Can you work these out from the model? Positions are in its coordinate system, mm. Give positions to 0.01 mm unless a question says otherwise; leave off trailing zeros. Loops run counter-clockwise (first coordinate to the right, second up) from the corner with the lowest first, then second, coordinate; pieces in that order, holes last. Notation, with made-up numbers: M -40,19 L -30,19 A24 ccw -30,57 Z; hole C 84,-17 d2. An arc over 180 degrees is marked long. Put each result on its own line as item: value. Start each with the question number.
1) Imagine slicing it at A-A (x = 231.5). Write out the boundary of the cut face in (y, z), then the cut area to 3 significant figures.
2) Please list where these lines run through material, in increasing order: line 1 along Z through (x, y) = (548, 40); line 2 along Z through (x, y) = (228, 70); line 3 along Y through (x, z) = (638, 6.5). Write a range as from..to.
3) Imagine slicing it at B-B (y = 31.5). Write out the boundary of the cut face in (x, z), then the cut area to 3 significant figures.
4) For P1, Ø5, axis at x = 317, y = 3, coming from the +Z side; P2, Ø6.5, axis at x = 681.5, z = 5, coming from the -Y side; P3, Ø6.5, axis at y = 66, z = 7.5, coming from the +X side, each with a flat end and sliding along its axis, tell me the tip position at first contact or that it passes through.
5) Imagine slicing it at C-C (z = 2.5). Write out the boundary of the cut face in (x, y), then the cut area to 3 significant figures.
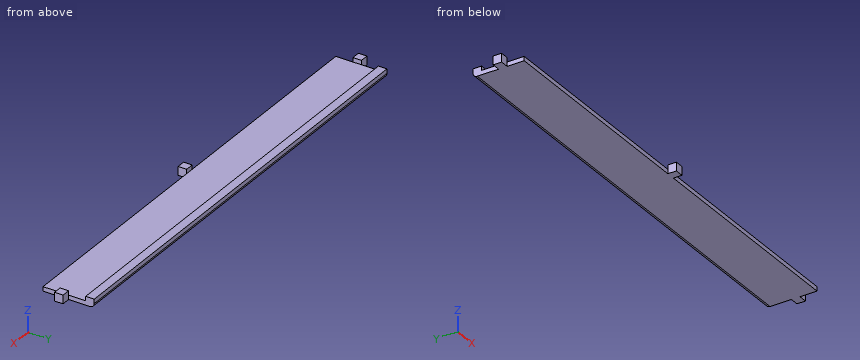
Autodesk Inventor part; units mm, degrees
ref_plane "YZ Plane" through (0, 0, 0) normal (1, 0, 0) x (0, 1, 0)
ref_plane "XZ Plane" through (0, 0, 0) normal (0, 1, 0) x (-1, 0, 0)
ref_plane "XY Plane" through (0, 0, 0) normal (0, 0, 1) x (1, 0, 0)
sketch "Sketch1" plane through (0, 0, 0) normal (0, 0, 1) x (1, 0, 0)
  line L0 (673.1, 76.2) -> (0, 76.2)
  line L1 (0, 25.4) -> (-12.7, 25.4)
  line L2 (-12.7, 25.4) -> (-12.7, 38.1)
  line L3 (-12.7, 38.1) -> (0, 38.1)
  line L4 (0, 76.2) -> (0, 38.1)
  line L5 (0, 25.4) -> (0, 0)
  line L6 (336.55, 12.7) -> (336.55, 76.2) construction
  line L7 (673.1, 25.4) -> (685.8, 25.4)
  line L8 (685.8, 25.4) -> (685.8, 38.1)
  line L9 (685.8, 38.1) -> (673.1, 38.1)
  line L10 (673.1, 0) -> (673.1, 25.4)
  line L11 (673.1, 38.1) -> (673.1, 76.2)
  line L12 (342.9, -12.7) -> (330.2, -12.7)
  line L13 (330.2, -12.7) -> (330.2, 0)
  line L14 (342.9, 0) -> (342.9, -12.7)
  line L15 (330.2, 0) -> (342.9, 0) construction
  line L16 (336.55, 0) -> (336.55, -12.7) construction
  line L17 (0, 0) -> (330.2, 0)
  line L18 (342.9, 0) -> (673.1, 0)
  point P0 (0, 34.925)
  point P1 (673.1, 34.925)
  dimension "d0" = 673.1
  dimension "d1" = 76.2
  dimension "d9" = 12.7
  dimension "d12" = 12.7
  dimension "d16" = 12.7
  dimension "d17" = 25.4
  dimension "d19" = 25.4
extrude "Extrusion1" add sketch "Sketch1" along normal blind 12.7
sketch "Sketch2" plane through (0, 0, 12.7) normal (0, 0, 1) x (1, 0, 0)
  line L0 (0, 0) -> (673.1, 0)
  line L1 (673.1, 0) -> (673.1, 63.5)
  line L2 (673.1, 63.5) -> (0, 63.5)
  line L3 (0, 63.5) -> (0, 0)
  dimension "d4" = 673.1
  dimension "d5" = 63.5
extrude "Extrusion2" cut sketch "Sketch2" against normal blind 6.35
fillet "Fillet1" radius 6.35 1 edges at (336.55, 76.2, 0)
equation "\"d19\" = d17"
properties part number "Arm Side" material "PVC-Piping"
Recorded:
1. outline: M 0,0 L 69.85,0 A6.35 ccw 76.2,6.35 L 76.2,12.7 L 63.5,12.7 L 63.5,6.35 L 0,6.35 Z
1. area: 556 mm²
2. line 1: 0..6.35
2. line 2: 0..12.7
2. line 3: 63.5..76.2
3. outline: M -12.7,0 L 685.8,0 L 685.8,12.7 L 673.1,12.7 L 673.1,6.35 L 0,6.35 L 0,12.7 L -12.7,12.7 Z
3. area: 4,600 mm²
4. P1: z = 6.35
4. P2: y = 25.4
4. P3: x = 673.1
5. outline: M -12.7,25.4 L 0,25.4 L 0,0 L 330.2,0 L 330.2,-12.7 L 342.9,-12.7 L 342.9,0 L 673.1,0 L 673.1,25.4 L 685.8,25.4 L 685.8,38.1 L 673.1,38.1 L 673.1,74.9 L 0,74.9 L 0,38.1 L -12.7,38.1 Z
5. area: 50,900 mm²
